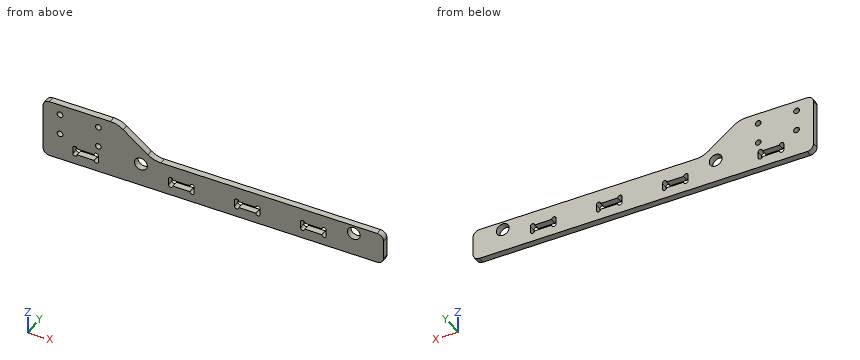
from build123d import *

# Parameters (mm, degrees)
SKETCH_1_W          = 160
SKETCH_1_H          = 15
EXTRUDE_1_DEPTH     = 3
EXTRUDE_2_DEPTH     = 3
SKETCH_3_W          = 12
SKETCH_3_H          = 3
CUT_EXTRUDE_1_DEPTH = 83.639276376
SKETCH_4_R          = 1
CUT_EXTRUDE_2_DEPTH = 83.639276376
CUT_EXTRUDE_4_DEPTH = 83.639276376
FILLET_1_R          = 3
FILLET_2_R          = 10
SKETCH_7_R          = 3
CUT_EXTRUDE_5_DEPTH = 83.639276376
SKETCH_8_R          = 1.35
CUT_EXTRUDE_6_DEPTH = 83.639276376


with BuildPart() as part:
    # 草图1 → 凸台-拉伸1 (new body)
    with BuildSketch(Plane(origin=(0, 0, 0), x_dir=(1, 0, 0), z_dir=(0, 1, 0))):
        Rectangle(SKETCH_1_W, SKETCH_1_H)
    extrude(amount=EXTRUDE_1_DEPTH)

    # 草图2 → 凸台-拉伸2 (add)
    with BuildSketch(Plane(origin=(0, 3, 0), x_dir=(1, 0, 0), z_dir=(0, 1, 0))):
        Polygon((-28, -7.5), (-80, -7.5), (-80, -20.5), (-45, -20.5), align=None)
    extrude(amount=-EXTRUDE_2_DEPTH)

    # 草图3 → 切除-拉伸1 (cut, through all)
    with BuildSketch(Plane.XZ):
        with Locations((16, -1)):
            Rectangle(SKETCH_3_W, SKETCH_3_H)
        with Locations((47, -1)):
            Rectangle(SKETCH_3_W, SKETCH_3_H)
        with Locations((-15, -1)):
            Rectangle(SKETCH_3_W, SKETCH_3_H)
        with Locations((-60, -1)):
            Rectangle(SKETCH_3_W, SKETCH_3_H)
    extrude(amount=-CUT_EXTRUDE_1_DEPTH, mode=Mode.SUBTRACT)

    # 草图4 → 切除-拉伸2 (cut, through all)
    with BuildSketch(Plane.XZ):
        with Locations((52, -2.5)):
            Circle(SKETCH_4_R)
        with Locations((42, -2.5)):
            Circle(SKETCH_4_R)
        with Locations((21, -2.5)):
            Circle(SKETCH_4_R)
        with Locations((11, -2.5)):
            Circle(SKETCH_4_R)
        with Locations((-10, -2.5)):
            Circle(SKETCH_4_R)
        with Locations((-20, -2.5)):
            Circle(SKETCH_4_R)
        with Locations((-65, -2.5)):
            Circle(SKETCH_4_R)
        with Locations((-55, -2.5)):
            Circle(SKETCH_4_R)
        with Locations((-55, 0.5)):
            Circle(SKETCH_4_R)
        with Locations((-65, 0.5)):
            Circle(SKETCH_4_R)
        with Locations((-20, 0.5)):
            Circle(SKETCH_4_R)
        with Locations((-10, 0.5)):
            Circle(SKETCH_4_R)
        with Locations((11, 0.5)):
            Circle(SKETCH_4_R)
        with Locations((21, 0.5)):
            Circle(SKETCH_4_R)
        with Locations((42, 0.5)):
            Circle(SKETCH_4_R)
        with Locations((52, 0.5)):
            Circle(SKETCH_4_R)
    extrude(amount=-CUT_EXTRUDE_2_DEPTH, mode=Mode.SUBTRACT)

    # 草图5 → 切除-拉伸4 (cut, through all)
    with BuildSketch(Plane.XZ):
        with BuildLine():
            Line((19.980196097, 0.52), (12.019803903, 0.52))
            ThreePointArc((12.019803903, 0.52), (10.989999519, 1.519950975), (9.98, 0.5))
            Line((9.98, 0.5), (9.98, -2.5))
            ThreePointArc((9.98, -2.5), (10.989999519, -3.519950975), (12.019803903, -2.52))
            Line((12.019803903, -2.52), (19.980196097, -2.52))
            ThreePointArc((19.980196097, -2.52), (21.010000481, -3.519950975), (22.02, -2.5))
            Line((22.02, -2.5), (22.02, 0.5))
            ThreePointArc((22.02, 0.5), (21.010000481, 1.519950975), (19.980196097, 0.52))
        make_face()
        with BuildLine():
            Line((53.02, -2.5), (53.02, 0.5))
            ThreePointArc((53.02, 0.5), (52.010000481, 1.519950975), (50.980196097, 0.52))
            Line((50.980196097, 0.52), (43.019803903, 0.52))
            ThreePointArc((43.019803903, 0.52), (41.989999519, 1.519950975), (40.98, 0.5))
            Line((40.98, 0.5), (40.98, -2.5))
            ThreePointArc((40.98, -2.5), (41.989999519, -3.519950975), (43.019803903, -2.52))
            Line((43.019803903, -2.52), (50.980196097, -2.52))
            ThreePointArc((50.980196097, -2.52), (52.010000481, -3.519950975), (53.02, -2.5))
        make_face()
        with BuildLine():
            Line((-11.019803903, 0.52), (-18.980196097, 0.52))
            ThreePointArc((-18.980196097, 0.52), (-20.010000481, 1.519950975), (-21.02, 0.5))
            Line((-21.02, 0.5), (-21.02, -2.5))
            ThreePointArc((-21.02, -2.5), (-20.010000481, -3.519950975), (-18.980196097, -2.52))
            Line((-18.980196097, -2.52), (-11.019803903, -2.52))
            ThreePointArc((-11.019803903, -2.52), (-9.989999519, -3.519950975), (-8.98, -2.5))
            Line((-8.98, -2.5), (-8.98, 0.5))
            ThreePointArc((-8.98, 0.5), (-9.989999519, 1.519950975), (-11.019803903, 0.52))
        make_face()
        with BuildLine():
            Line((-66.02, -2.5), (-66.02, 0.5))
            ThreePointArc((-66.02, 0.5), (-65.010000481, 1.519950975), (-63.980196097, 0.52))
            Line((-63.980196097, 0.52), (-56.019803903, 0.52))
            ThreePointArc((-56.019803903, 0.52), (-54.989999519, 1.519950975), (-53.98, 0.5))
            Line((-53.98, 0.5), (-53.98, -2.5))
            ThreePointArc((-53.98, -2.5), (-54.989999519, -3.519950975), (-56.019803903, -2.52))
            Line((-56.019803903, -2.52), (-63.980196097, -2.52))
            ThreePointArc((-63.980196097, -2.52), (-65.010000481, -3.519950975), (-66.02, -2.5))
        make_face()
    extrude(amount=-CUT_EXTRUDE_4_DEPTH, mode=Mode.SUBTRACT)

    # 圆角1
    fillet_1_edges = [part.edges().sort_by_distance(p)[0] for p in [
        (-80, 1.5, 20.5),
        (80, 1.5, 7.5),
        (-80, 1.5, -7.5),
        (80, 1.5, -7.5),
    ]]
    fillet(fillet_1_edges, radius=FILLET_1_R)

    # 圆角2
    fillet_2_edges = [part.edges().sort_by_distance(p)[0] for p in [
        (-28, 1.5, 7.5),
        (-45, 1.5, 20.5),
    ]]
    fillet(fillet_2_edges, radius=FILLET_2_R)

    # 草图7 → 切除-拉伸5 (cut, through all)
    with BuildSketch(Plane.XZ):
        with Locations(Location((66, 3.5, 0), (0, 0, 270))):
            Circle(SKETCH_7_R)
        with Locations(Location((-34, 3.5, 0), (0, 0, 270))):
            Circle(SKETCH_7_R)
    extrude(amount=-CUT_EXTRUDE_5_DEPTH, mode=Mode.SUBTRACT)

    # 草图8 → 切除-拉伸6 (cut, through all)
    with BuildSketch(Plane.XZ):
        with Locations(Location((-72, 5.5, 0), (0, 0, 270))):
            Circle(SKETCH_8_R)
        with Locations(Location((-72, 15.5, 0), (0, 0, 90))):
            Circle(SKETCH_8_R)
        with Locations(Location((-54, 15.5, 0), (0, 0, 270))):
            Circle(SKETCH_8_R)
        with Locations(Location((-54, 5.5, 0), (0, 0, 90))):
            Circle(SKETCH_8_R)
    extrude(amount=-CUT_EXTRUDE_6_DEPTH, mode=Mode.SUBTRACT)


solid = part.part
Read the model definition and answer for the solid it produces. Units are mm, in the model's axes. Give positions to 0.01 mm unless a question says otherwise; leave off trailing zeros. Write each loop counter-clockwise with the first axis right and the second up, starting at its lowest first coordinate (ties: lowest second). Pieces come first, ordered by that corner, then holes. Notation, with made-up numbers: (1.25, -14) - (50.25, -14) arc R26 cw to (50.25, 21) - close; hole circle Ø1 at (22, 85.5). An arc over 180 degrees is marked (long way). Use CSV: the item, a comma, the result in double quotes. Start each with the question number.
(1) Find section A-A (x = -72). Give the vertices of the cut face in (y, z), plus the area to 3 significant figures.
(2) Find section C-C (y = 1.05). Count the separate pieces of the cut face and the enclosed holes in it, plus the area to 3 significant figures.
(3) Find section D-D (x = 49.5). Give the vertices of the cut face in (y, z).
(4) Consider line 1 along Z through (x, y) = (-72, 1.3); line 2 along X through (y, z) = (1.5, 3.5); line 3 along X through (y, z) = (2.8, 0.25). Determine where each line is inside the solid, lowest interval first.
(5) Find section B-B (x = 66). Give the vertices of the cut face in (y, z).
Findings below:
1,outline,"(0, -7.5) - (3, -7.5) - (3, 4.15) - (0, 4.15) - close; (0, 6.85) - (3, 6.85) - (3, 14.15) - (0, 14.15) - close; (0, 16.85) - (3, 16.85) - (3, 20.5) - (0, 20.5) - close"
1,area,"67.8 mm2"
2,separate pieces,"1"
2,enclosed holes,"10"
2,area,"2,710 mm2"
3,outline,"(0, -7.5) - (3, -7.5) - (3, -2.52) - (0, -2.52) - close; (0, 0.52) - (3, 0.52) - (3, 7.5) - (0, 7.5) - close"
4,line 1,"-7.5 to 4.15, 6.85 to 14.15, 16.85 to 20.5"
4,line 2,"-80 to -37, -31 to 63, 69 to 80"
4,line 3,"-80 to -66.02, -53.98 to -21.02, -8.98 to 9.98, 22.02 to 40.98, 53.02 to 80"
5,outline,"(0, -7.5) - (3, -7.5) - (3, 0.5) - (0, 0.5) - close; (0, 6.5) - (3, 6.5) - (3, 7.5) - (0, 7.5) - close"
